from build123d import *

# Parameters (mm, degrees)
AXLE_SUPPORT_PLATE_R = 7.030128061
AXLE_SUPPORT_PLATE_W = 6.35
AXLE_SUPPORT_PLATE_H = 6.35
BOSS_EXTRUDE1_DEPTH  = 6.35


with BuildPart() as part:
    # Axle Support Plate → Boss-Extrude1 (new body)
    with BuildSketch(Plane(origin=(0, 0, 0), x_dir=(1, 0, 0), z_dir=(0, 1, 0))):
        Polygon((31.160128061, -169.56756403), (31.160128061, 169.56756403), (0, 169.56756403), (0, -175.91756403), (6.35, -175.91756403), (6.35, -169.56756403), (12.7, -169.56756403), (12.7, -175.91756403), (19.05, -175.91756403), (19.05, -169.56756403), align=None)
        with Locations(Location((19.05, 157.45743597, 0), (0, 0, 270))):
            Circle(AXLE_SUPPORT_PLATE_R, mode=Mode.SUBTRACT)
        with Locations(Location((19.05, -134.64256403, 0), (0, 0, 90))):
            Circle(AXLE_SUPPORT_PLATE_R, mode=Mode.SUBTRACT)
        with Locations((9.525, -92.075)):
            Rectangle(AXLE_SUPPORT_PLATE_W, AXLE_SUPPORT_PLATE_H, mode=Mode.SUBTRACT)
        with Locations((9.525, 92.075)):
            Rectangle(AXLE_SUPPORT_PLATE_W, AXLE_SUPPORT_PLATE_H, mode=Mode.SUBTRACT)
    extrude(amount=BOSS_EXTRUDE1_DEPTH)


solid = part.part
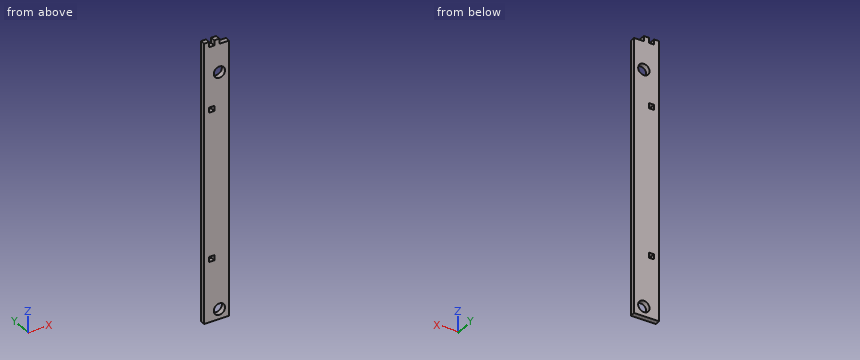
Read the model definition and answer for the solid it produces. Units are mm, in the model's axes. Give positions to 0.01 mm unless a question says otherwise; leave off trailing zeros. Loops run counter-clockwise (first coordinate to the right, second up) from the corner with the lowest first, then second, coordinate; pieces in that order, holes last. Notation, with made-up numbers: (-23.75, 49.5) -> (11.25, 49.5) arc R28 ccw to (11.25, 86.5) -> close; hole circle Ø6 at (-14.5, 41.5). An arc over 180 degrees is marked (long way). Use a Markdown table: item, result.
Q1. Section B-B, the plane x = 16 is taken. Determine the outline of the cut face in (y, z), then the cut area to 3 significant figures.
Solved:
| item | result |
|---|---|
| outline | (0, -169.57) -> (6.35, -169.57) -> (6.35, -163.79) -> (0, -163.79) -> close; (0, -151.12) -> (6.35, -151.12) -> (6.35, 128.31) -> (0, 128.31) -> close; (0, 140.98) -> (6.35, 140.98) -> (6.35, 175.92) -> (0, 175.92) -> close |
| area | 2,030 mm^2 |
Q2. Find the intervals of material crossed by line 1 along Z through (x, y) = (10, 4.25); line 2 along Z through (x, y) = (16.5, 6); line 3 along X through (y, z) = (3.5, 137), in increasing order.
Solved:
| item | result |
|---|---|
| line 1 | z = -169.57 to -95.25, -88.9 to 88.9, 95.25 to 169.57 |
| line 2 | z = -169.57 to -164.01, -150.91 to 128.09, 141.19 to 175.92 |
| line 3 | x = 0 to 12.43, 25.67 to 31.16 |
Q3. Each of these flat-tipped pins is pushed along its axis until it touches: pin 1 (3 mm diameter, centred on x = 21, y = 5.5, fed in from +Z); pin 2 (11 mm diameter, centred on x = 19.05, z = 134.64, fed in from -Y). Where does it stop, or does it pass through?
Solved:
| item | result |
|---|---|
| pin 1 | stops at z = 169.57 |
| pin 2 | passes through |
Q4. Section A-A, the plane y = 3.75 is taken. Determine the outline of the cut face in (x, z), then the cut area to 3 significant figures.
Solved:
| item | result |
|---|---|
| outline | (0, -169.57) -> (31.16, -169.57) -> (31.16, 169.57) -> (19.05, 169.57) -> (19.05, 175.92) -> (12.7, 175.92) -> (12.7, 169.57) -> (6.35, 169.57) -> (6.35, 175.92) -> (0, 175.92) -> close; hole (6.35, -95.25) -> (12.7, -95.25) -> (12.7, -88.9) -> (6.35, -88.9) -> close; hole (6.35, 88.9) -> (12.7, 88.9) -> (12.7, 95.25) -> (6.35, 95.25) -> close; hole circle Ø14.06 at (19.05, -157.46); hole circle Ø14.06 at (19.05, 134.64) |
| area | 10,300 mm^2 |
